```python
from build123d import *

# Parameters (mm, degrees)
F1_DEPTH = 25
F2_R     = 33.4969963506
F2_R_2   = 31.5
F3_DEPTH = 3
F4_R     = 10.9661073878
F5_DEPTH = 25
F6_DEPTH = 22
F7_DEPTH = 25


with BuildPart() as f1:
    # F0 (on Top) → F1 (new body)
    with BuildSketch(Plane.XY):
        with BuildLine():
            ThreePointArc((53.7871589783, 22.7454871565), (53.8780832708, 23.694684553), (54.1475492573, 24.6093599089))
            ThreePointArc((54.1475492573, 24.6093599089), (53.3520531244, 32.0716472029), (46.7241737037, 35.5915563126))
            Line((46.7241737037, 35.5915563126), (-49.3051404481, 35.5915563126))
            ThreePointArc((-49.3051404481, 35.5915563126), (-51.824342213, 34.910540275), (-53.6572972564, 33.0530052997))
            ThreePointArc((-53.6572972564, 33.0530052997), (-43.5514249028, -21.6702688765), (-3.3649580648, -60.1645967141))
            Line((-3.3649580648, -60.1645967141), (-0.9160143624, -60.9986215442))
            ThreePointArc((-0.9160143624, -60.9986215442), (4.2266959979, -62.32076541), (9.0644102401, -60.1316890835))
            Line((9.0644102401, -60.1316890835), (40.2996465564, -23.2034455985))
            ThreePointArc((40.2996465564, -23.2034455985), (43.1207673401, -20.3529292947), (44.5950298413, -16.6232221009))
            Line((44.5950298413, -16.6232221009), (53.7871589783, 22.7454871565))
        make_face()
        with BuildLine():
            ThreePointArc((8.563389259, -56.098732374), (2.6455954518, -59.6001717259), (-1.7897081955, -54.3457980587))
            Line((-1.7897081955, -54.3457980587), (-1.775094173, -45.4805905471))
            ThreePointArc((-1.775094173, -45.4805905471), (3.9099702523, -41.0468470679), (8.7971219068, -46.3472043639))
            Line((8.7971219068, -46.3472043639), (8.563389259, -56.098732374))
        make_face(mode=Mode.SUBTRACT)
        with BuildLine():
            ThreePointArc((0, 31.5), (22.2738636074, 22.2738636074), (31.5, 0))
            ThreePointArc((31.5, 0), (22.0210780969, -22.5238122762), (-0.7109282192, -31.4919764554))
            ThreePointArc((-0.7109282192, -31.4919764554), (-2.2037245281, -31.4228197049), (-3.6915609888, -31.282940678))
            ThreePointArc((-3.6915609888, -31.282940678), (-31.4949418681, 0.5644791617), (-2.5681911856, 31.3951332858))
            ThreePointArc((-2.5681911856, 31.3951332858), (-1.2851656502, 31.4737724026), (0, 31.5))
        make_face(mode=Mode.SUBTRACT)
        with BuildLine():
            ThreePointArc((-48.8032426669, 22.148864889), (-49.7645237359, 27.1276520058), (-45.0716722429, 29.0484662373))
            Line((-45.0716722429, 29.0484662373), (-36.743987983, 24.4311855453))
            ThreePointArc((-36.743987983, 24.4311855453), (-35.2015648727, 18.9642062238), (-40.6811828695, 17.4673032339))
            Line((-40.6811828695, 17.4673032339), (-48.8032426669, 22.148864889))
        make_face(mode=Mode.SUBTRACT)
        with BuildLine():
            ThreePointArc((41.2858330553, 19.7592478666), (35.7800785258, 21.1569599304), (37.223531508, 26.6508998136))
            Line((37.223531508, 26.6508998136), (45.3389127294, 31.3440291017))
            ThreePointArc((45.3389127294, 31.3440291017), (50.131309387, 29.6871293693), (49.448357561, 24.6625936444))
            Line((49.448357561, 24.6625936444), (41.2858330553, 19.7592478666))
        make_face(mode=Mode.SUBTRACT)
    extrude(amount=F1_DEPTH)

    # F2 (on face) → F3 (join)
    with BuildSketch(Plane(origin=(0, 0, 0), x_dir=(1, 0, 0), z_dir=(0, 0, -1))):
        Circle(F2_R)
        Circle(F2_R_2, mode=Mode.SUBTRACT)
        Circle(F2_R_2)
    extrude(amount=-F3_DEPTH)

    # F4 (on face) → F5 (cut)
    with BuildSketch(Plane.XY.offset(3)):
        with Locations((16.1272473633, 0)):
            Circle(F4_R)
    extrude(amount=-F5_DEPTH, mode=Mode.SUBTRACT)

    # F4 (on face) → F6 (join)
    with BuildSketch(Plane.XY.offset(3)):
        with BuildLine():
            ThreePointArc((26.4328128914, 17.1334877549), (22.8210045885, 13.9789914635), (18.2305140411, 12.5921235522))
            ThreePointArc((18.2305140411, 12.5921235522), (3.48568477, -1.7821900775), (21.6297892683, -11.5198671371))
            ThreePointArc((21.6297892683, -11.5198671371), (25.4383279787, -11.3846100228), (29.2333080601, -11.7330175088))
            ThreePointArc((29.2333080601, -11.7330175088), (32.5859089375, 3.1613345542), (26.4328128914, 17.1334877549))
        make_face()
        with Locations((16.1272473633, 0)):
            Circle(F4_R, mode=Mode.SUBTRACT)
    extrude(amount=F6_DEPTH)

    # F0 (on Top) → F7 (join)
    with BuildSketch(Plane.XY):
        with BuildLine():
            Line((-0.7109282192, -31.4919764554), (0, 31.5))
            ThreePointArc((0, 31.5), (-1.2851656502, 31.4737724026), (-2.5681911856, 31.3951332858))
            Line((-2.5681911856, 31.3951332858), (-3.6915609888, -31.282940678))
            ThreePointArc((-3.6915609888, -31.282940678), (-2.2037245281, -31.4228197049), (-0.7109282192, -31.4919764554))
        make_face()
    extrude(amount=F7_DEPTH)


solid = f1.part
```
Work out the finished part from the listing and answer in its coordinate system (mm). A direction names the side the tool comes from. Give positions to 0.01 mm unless a question says otherwise; leave off trailing zeros. Order: outer loops, then holes, each group sorted by start corner. A loop starts at its lowest first (then second) coordinate and runs counter-clockwise, first axis right, second up. Notation, with made-up numbers: (77, -11) - (89, -11) arc R19 ccw to (89, 7) - close; hole circle Ø5 at (61.5, 53.5). An arc over 180 degrees is marked (long way). One line per item, written item: value. Start each with the question number.
1. Section D-D, the plane y = -35.5 is taken. Write down the section's boundary in (x, z), then the cut area to 3 significant figures.
2. Section A-A, the plane y = 0 is taken. Write down the section's boundary in (x, z).
3. Each of these flat-tipped pins is pushed along its axis until it touches: pin 1 Ø8 at (y, z) = (-10.5, 11.5) entering from +X; pin 2 Ø6 at (x, z) = (-36.5, 12) entering from -Y; pin 3 Ø1 at (y, z) = (-52.5, 9) entering from +X. Where does it stop, or does it pass through?
4. Which of the six approach directions +Z, -Z, +X, -X, +Y, -Y give full straight-line access (tool end or side, diameter ignored) to faces 1 (the face through (53.4, 32, 12.3)), 2 (the face through (3.8, -41.04, 12.32)), 3 (the face through (22.88, 14.01, 13.85))?
5. For a pull along X with two mould halves and no side action, classify faces 4 (the face through (43.09, -20.4, 12.32)), 5 (the face through (-2.158, -60.576, 12.325)), 6 (the face through (-44.69, 19.78, 12.32)) as released by +X, released by -X, zero draft, split by the parting line, or undercut.
6. Section B-B, the plane z = 10.5 is taken. Count the separate pieces of the cut face and the enclosed holes in it, then the cut area to 3 significant figures.
7. Consider line 1 (Y direction, x = 19, z = 23.5); line 2 (X direction, y = 24.5, z = 19.5); line 3 (X direction, y = 5.5, z = 20). Determine where each line is inside the solid, lowest interval first.
8. Section C-C, the plane x = 16.5 is taken. Write down the section's boundary in (y, z).
Filled sheet:
1. outline: (-34.36, 0) - (29.9, 0) - (29.9, 25) - (-34.36, 25) - close
1. area: 1,610 mm²
2. outline: (-51.86, 0) - (5.16, 0) - (5.16, 25) - (3.36, 25) - (3.36, 3) - (-0.36, 3) - (-0.36, 25) - (-3.13, 25) - (-3.13, 3) - (-31.5, 3) - (-31.5, 25) - (-51.86, 25) - close; (27.09, 0) - (48.48, 0) - (48.48, 25) - (27.09, 25) - close
3. pin 1: x = 46.96
3. pin 2: y = -36.55
3. pin 3: x = 15.94
4. face 1: +Z, -Z, +X
4. face 2: +Z, -Z
4. face 3: +Z
5. face 4: released by +X
5. face 5: released by -X
5. face 6: undercut
6. separate pieces: 1
6. enclosed holes: 6
6. area: 4,760 mm²
7. line 1: -48.39 to -25.12, -12.44 to -10.58, 10.58 to 12.68, 25.12 to 35.59
7. line 2: -54.36 to -50.18, -36.87 to -19.8, -2.69 to -0.08, 19.8 to 35.45, 49.18 to 54.11
7. line 3: -53.02 to -31.02, -3.03 to -0.29, 4.61 to 6.64, 25.61 to 49.76
8. outline: (-51.34, 0) - (-10.96, 0) - (-10.96, 25) - (-12.76, 25) - (-12.76, 3) - (-26.83, 3) - (-26.83, 25) - (-51.34, 25) - close; (10.96, 0) - (35.59, 0) - (35.59, 25) - (26.83, 25) - (26.83, 3) - (12.76, 3) - (12.76, 25) - (10.96, 25) - close
